The model under review builds one solid part; all positions refer to its coordinate system, in mm. A direction names the side the tool comes from. Give positions to 0.01 mm unless a question says otherwise; leave off trailing zeros. Order: outer loops, then holes, each group sorted by start corner. A loop starts at its lowest first (then second) coordinate and runs counter-clockwise, first axis right, second up. Notation, with made-up numbers: (83.5, -30) - (95.5, -30) arc R25 ccw to (95.5, 8) - close; hole circle Ø5 at (61.5, 23.5). An arc over 180 degrees is marked (long way). Write item = value, one per line. Start each with the question number.
1. We need section A-A, the plane y = 15.5. Give the boundary of the cut face in (x, z).
2. Machinability: for faces 1 (the flat face through (-166, 66.654, -32)), 2 (the cylindrical face through (-193.82, 67.47, -43.19)), 3 (the flat face through (-183.376, 53.8, 0.4)), which of the approach directions +Z, -Z, +X, -X, +Y, -Y give a long, thin tool a straight path to every point of the face, cutting with its end or side? Answer none if there is none.
3. Wall thickness on probe 1 along Y at (x, z) = (-163, -41); probe 2 along Z at (x, y) = (-187.5, -16.5): over which ranges is each line inside the solid? List them lowest first.
4. For P1, Ø5.5, axis at x = -190.13, y = 43.9, coming from the -Z side; P2, Ø0.8, axis at y = -55.5, z = 1, coming from the +X side; P3, Ø12, axis at x = -124, z = -27.5, coming from the -Y side, all flat-tipped, find the tip position at first contact; note any pin that passes through.
5. We need section B-B, the plane x = -154.5. Give the boundary of the cut face in (y, z), and give its area (3 significant figures).
6. Mouldability with a two-part tool opening along Y and no side actions: class faces 4 (the flat face through (-190, -2, -0.1)), 5 (the cylindrical face through (-192.17, -56.57, 0.69)), 6 (the flat face through (-166, 68.254, -32)) as pulls with the +Y half, pulls with the -Y half, needs draft (parallel to the pull), parting line crosses it, or undercut.
from build123d import *

# Parameters (mm, degrees)
SKETCH1_R                    = 2.0447
BOSS_EXTRUDE1_DEPTH          = 1.5
CONVERT_SOLID1_START         = -0.100000102
CONVERT_SOLID1_OUTLINE_R     = 2.0447
CONVERT_SOLID1_DEPTH         = 0.100000102
EDGE_FLANGE1_STRIP_W         = 26.400000408
EDGE_FLANGE1_STRIP_H         = 1.600000102
EDGE_FLANGE1_STRIP_CUT_DEPTH = 13.5
EDGE_FLANGE1_DEPTH           = 13.5
EDGE_FLANGE1_FLAT_DEPTH      = 1.600000102
CUT_EXTRUDE1_DEPTH           = 241.95509557
CUT_EXTRUDE1_DEPTH_BACK      = 3.81
SKETCH14_R                   = 6.583720687


# Read off the part's stored shape, not the designer's step: Convert-Solid1
# Sheet-metal steps are written as plain solids
with BuildPart() as part:
    # Sketch1 → Boss-Extrude1 (new body)
    with BuildSketch(Plane.XY):
        with BuildLine():
            Line((-183.376451986, -43.514598677), (-183.376451986, -62.800541688))
            Line((-183.376451986, -62.800541688), (-196.876451986, -62.800541688))
            Line((-196.876451986, -62.800541688), (-196.876451986, 68.254211442))
            Line((-196.876451986, 68.254211442), (-183.376451986, 68.254211442))
            Line((-183.376451986, 68.254211442), (-183.376451986, 47.120607659))
            Line((-183.376451986, 47.120607659), (-183.376451986, 40.670801349))
            Line((-183.376451986, 40.670801349), (-183.376451986, 30.753207577))
            ThreePointArc((-183.376451986, 30.753207577), (-184.376452018, 27.528304422), (-183.376451986, 24.303401267))
            Line((-183.376451986, 24.303401267), (-183.376451986, 8.147207521))
            ThreePointArc((-183.376451986, 8.147207521), (-184.376451986, 4.922304422), (-183.376451986, 1.697401323))
            Line((-183.376451986, 1.697401323), (-183.376451986, -14.458792479))
            ThreePointArc((-183.376451986, -14.458792479), (-184.376451986, -17.683695578), (-183.376451986, -20.908598677))
            Line((-183.376451986, -20.908598677), (-183.376451986, -37.064792479))
            ThreePointArc((-183.376451986, -37.064792479), (-184.376451986, -40.289695578), (-183.376451986, -43.514598677))
        make_face()
        with Locations((-190.126451986, -56.65709566)):
            Circle(SKETCH1_R, mode=Mode.SUBTRACT)
        with Locations((-190.126451986, 43.895704504)):
            Circle(SKETCH1_R, mode=Mode.SUBTRACT)
    extrude(amount=BOSS_EXTRUDE1_DEPTH)

    # Convert-Solid1 outline → Convert-Solid1 (add)
    with BuildSketch(Plane.XY.offset(CONVERT_SOLID1_START)):
        with BuildLine():
            Line((-183.376451986, -62.800541688), (-183.376451986, -43.514598677))
            ThreePointArc((-183.376451986, -43.514598677), (-184.376451986, -40.289695578), (-183.376451986, -37.064792479))
            Line((-183.376451986, -37.064792479), (-183.376451986, -20.908598677))
            ThreePointArc((-183.376451986, -20.908598677), (-184.376451986, -17.683695578), (-183.376451986, -14.458792479))
            Line((-183.376451986, -14.458792479), (-183.376451986, 1.697401323))
            ThreePointArc((-183.376451986, 1.697401323), (-184.376451986, 4.922304422), (-183.376451986, 8.147207521))
            Line((-183.376451986, 8.147207521), (-183.376451986, 24.303401267))
            ThreePointArc((-183.376451986, 24.303401267), (-184.376452018, 27.528304422), (-183.376451986, 30.753207577))
            Line((-183.376451986, 30.753207577), (-183.376451986, 68.254211442))
            Line((-183.376451986, 68.254211442), (-196.876451986, 68.254211442))
            Line((-196.876451986, 68.254211442), (-196.876451986, -62.800541688))
            Line((-196.876451986, -62.800541688), (-183.376451986, -62.800541688))
        make_face()
        with Locations((-190.126451986, -56.65709566)):
            Circle(CONVERT_SOLID1_OUTLINE_R, mode=Mode.SUBTRACT)
        with Locations((-190.126451986, 43.895704504)):
            Circle(CONVERT_SOLID1_OUTLINE_R, mode=Mode.SUBTRACT)
    extrude(amount=CONVERT_SOLID1_DEPTH)

    # Edge-Flange1 strip (across the edge) → Edge-Flange1 strip cut (cut)
    with BuildSketch(Plane(origin=(-196.876451986, 68.254211442, -0.100000102), x_dir=(0, -1, 0), z_dir=(1, 0, 0))):
        with Locations((-1.600000102, -0.800000051)):
            Rectangle(EDGE_FLANGE1_STRIP_W, EDGE_FLANGE1_STRIP_H)
    extrude(amount=EDGE_FLANGE1_STRIP_CUT_DEPTH, mode=Mode.SUBTRACT)

    # Edge-Flange1 bend section (across the edge) → Edge-Flange1 (add)
    with BuildSketch(Plane(origin=(-196.876451986, 68.254211442, -0.100000102), x_dir=(0, -1, 0), z_dir=(1, 0, 0))):
        with BuildLine():
            Line((0, 10), (1.600000102, 10))
            ThreePointArc((1.600000102, 10), (4.52893229, 2.928932188), (11.600000102, 0))
            Line((11.600000102, 0), (11.600000102, -1.600000102))
            ThreePointArc((11.600000102, -1.600000102), (3.397561368, 1.797561266), (0, 10))
        make_face()
    extrude(amount=EDGE_FLANGE1_DEPTH)

    # Edge-Flange1 profile (on flange) → Edge-Flange1 flat (add)
    with BuildSketch(Plane(origin=(0, 68.254211442, -0.100000102), x_dir=(1, 0, 0), z_dir=(0, 1, 0))):
        with BuildLine():
            Line((-196.876451986, 10), (-183.376451986, 10))
            Line((-183.376451986, 10), (-183.376451986, 19.305702381))
            ThreePointArc((-183.376451986, 19.305702381), (-180.400656883, 26.489907277), (-173.216451986, 29.465702381))
            Line((-173.216451986, 29.465702381), (-114.796451986, 29.465702381))
            Line((-114.796451986, 29.465702381), (-114.796451986, 45.983320267))
            Line((-114.796451986, 45.983320267), (-175.756451986, 45.983320267))
            Line((-175.756451986, 45.983320267), (-186.716451986, 45.983320267))
            ThreePointArc((-186.716451986, 45.983320267), (-193.900656883, 43.007525164), (-196.876451986, 35.823320267))
            Line((-196.876451986, 35.823320267), (-196.876451986, 10))
        make_face()
    extrude(amount=-EDGE_FLANGE1_FLAT_DEPTH)

    # Sketch14 → Cut-Extrude1 (cut, two sides: drawn at the far end of the back side and taken through both)
    with BuildSketch(Plane(origin=(0, 68.254211442, 0), x_dir=(1, 0, 0), z_dir=(0, 1, 0)).offset(-CUT_EXTRUDE1_DEPTH_BACK)):
        with Locations((-99.147079888, 65.798432199)):
            Circle(SKETCH14_R)
    extrude(amount=CUT_EXTRUDE1_DEPTH + CUT_EXTRUDE1_DEPTH_BACK, mode=Mode.SUBTRACT)


solid = part.part
Model answer:
q1.outline = (-196.88, -0.1) - (-183.38, -0.1) - (-183.38, 1.5) - (-196.88, 1.5) - close
q2.face_1 = -Z, +X, -X, -Y
q2.face_2 = -Z, -X, +Y, -Y
q2.face_3 = +Z, +X, +Y, -Y
q3.probe_1 = 66.65 to 68.25
q3.probe_2 = -0.1 to 1.5
q4.P1 = -0.1
q4.P2 = -183.38
q4.P3 = 66.65
q5.outline = (66.65, -46.08) - (68.25, -46.08) - (68.25, -29.57) - (66.65, -29.57) - close
q5.area = 26.4 mm2
q6.face_4 = needs draft
q6.face_5 = undercut
q6.face_6 = pulls with the +Y half
